Geometry check sheet. Reference: drawing and pictorial views, mm from the part's lowest x, y, z. A direction names the side the tool comes from. Give positions to 0.01 mm unless a question says otherwise; leave off trailing zeros. Order: outer loops, then holes, each group sorted by start corner. A loop starts at its lowest first (then second) coordinate and runs counter-clockwise, first axis right, second up. Notation, with made-up numbers: M 14.5,-37.5 L 41.5,-37.5 A35 ccw 41.5,-4.5 Z; hole C 2.5,10.25 d3. An arc over 180 degrees is marked long. Answer as CSV lines item,"result". Start each with the question number.
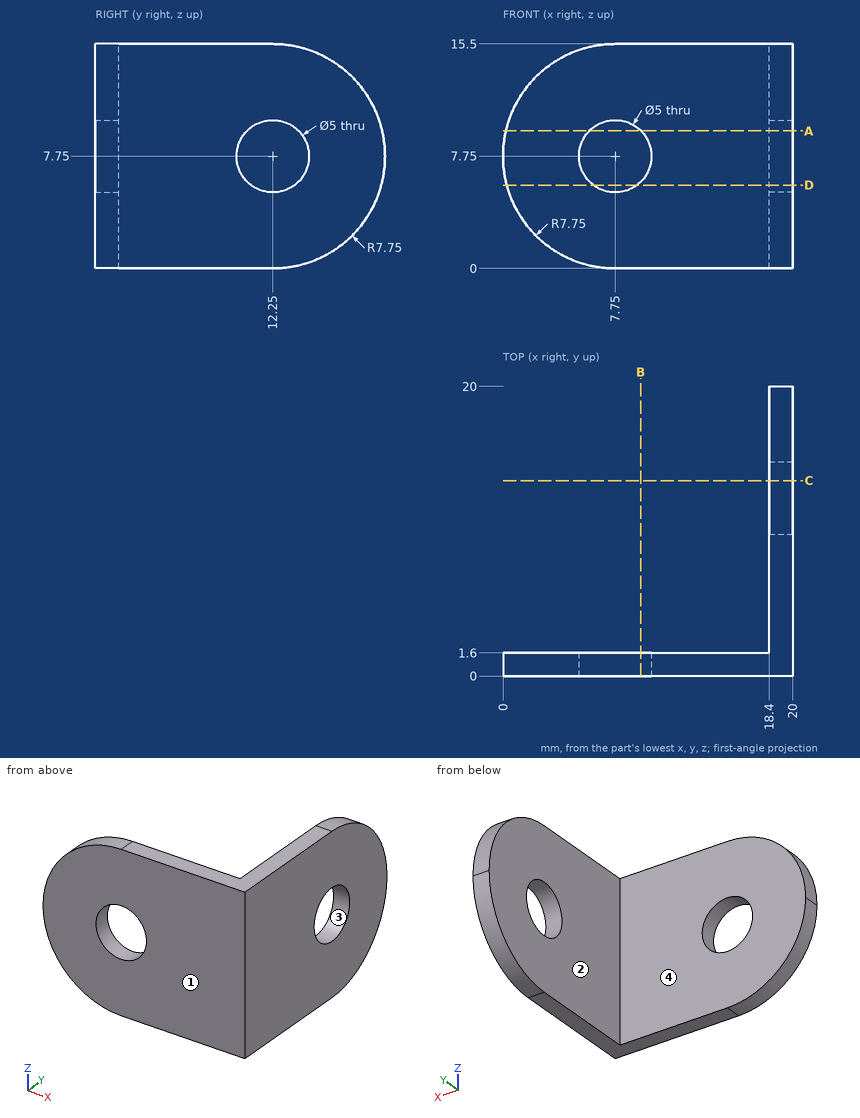
Item 1: Section check B-B on x = 9.5. Record the boundary of the cut face in (y, z), then the cut area to 3 significant figures.
Item 2: Section check C-C on y = 13.5. Record the boundary of the cut face in (x, z).
Item 3: Draft check along Z on the marked faces 3 and 4. Enter one of: pulls with the +Z half, pulls with the -Z half, needs draft (parallel to the pull), parting line crosses it, or undercut.
Item 4: Scan lines: line 1 along Z through (x, y) = (7.75, 0.55); line 2 along Y through (x, z) = (11.75, 9.75); line 3 along X through (y, z) = (4, 1.75). Record each from-to range of solid material in increasing order.
Item 5: Section check D-D on z = 5.75. Record the boundary of the cut face in (x, y).
Item 6: Access from +Z, -Z, +X, -X, +Y, -Y to the whole of each face (thin tool, end or side, straight path). Record for the marked faces 1 and 2.
Item 7: Depth check by flat-ended pin: pin 1 Ø2 at (x, z) = (6, 6.5) entering from +Y; pin 2 Ø3 at (y, z) = (9.5, 6) entering from -X. Enter the tip coordinate at first touch or a pass-through.
Item 8: Section check A-A on z = 9.5. Record the boundary of the cut face in (x, y), then the cut area to 3 significant figures.
Numbers:
1,outline,"M 0,0 L 1.6,0 L 1.6,5.96 L 0,5.96 Z; M 0,9.54 L 1.6,9.54 L 1.6,15.5 L 0,15.5 Z"
1,area,"19.1 mm2"
2,outline,"M 18.4,0.1 L 20,0.1 L 20,5.58 L 18.4,5.58 Z; M 18.4,9.92 L 20,9.92 L 20,15.4 L 18.4,15.4 Z"
3,face 3,"undercut"
3,face 4,"needs draft"
4,line 1,"0 to 5.25, 10.25 to 15.5"
4,line 2,"0 to 1.6"
4,line 3,"18.4 to 20"
5,outline,"M 0.26,0 L 6.25,0 L 6.25,1.6 L 0.26,1.6 Z; M 9.25,0 L 20,0 L 20,10.75 L 18.4,10.75 L 18.4,1.6 L 9.25,1.6 Z; M 18.4,13.75 L 20,13.75 L 20,19.74 L 18.4,19.74 Z"
6,face 1,"+Z, -Z, +X, -X, -Y"
6,face 2,"+Z, -Z, -X, +Y"
7,pin 1,"y = 1.6"
7,pin 2,"x = 18.4"
8,outline,"M 0.2,0 L 5.96,0 L 5.96,1.6 L 0.2,1.6 Z; M 9.54,0 L 20,0 L 20,10.46 L 18.4,10.46 L 18.4,1.6 L 9.54,1.6 Z; M 18.4,14.04 L 20,14.04 L 20,19.8 L 18.4,19.8 Z"
8,area,"49.4 mm2"
